Answer from the drawing. Dimensions are ordinates in mm from the lowest x, y and z of the part. A direction names the side the tool comes from. Round coordinates to 2 decimals unless told otherwise and drop trailing zeros. Order: outer loops, then holes, each group sorted by start corner. A loop starts at its lowest first (then second) coordinate and runs counter-clockwise, first axis right, second up.
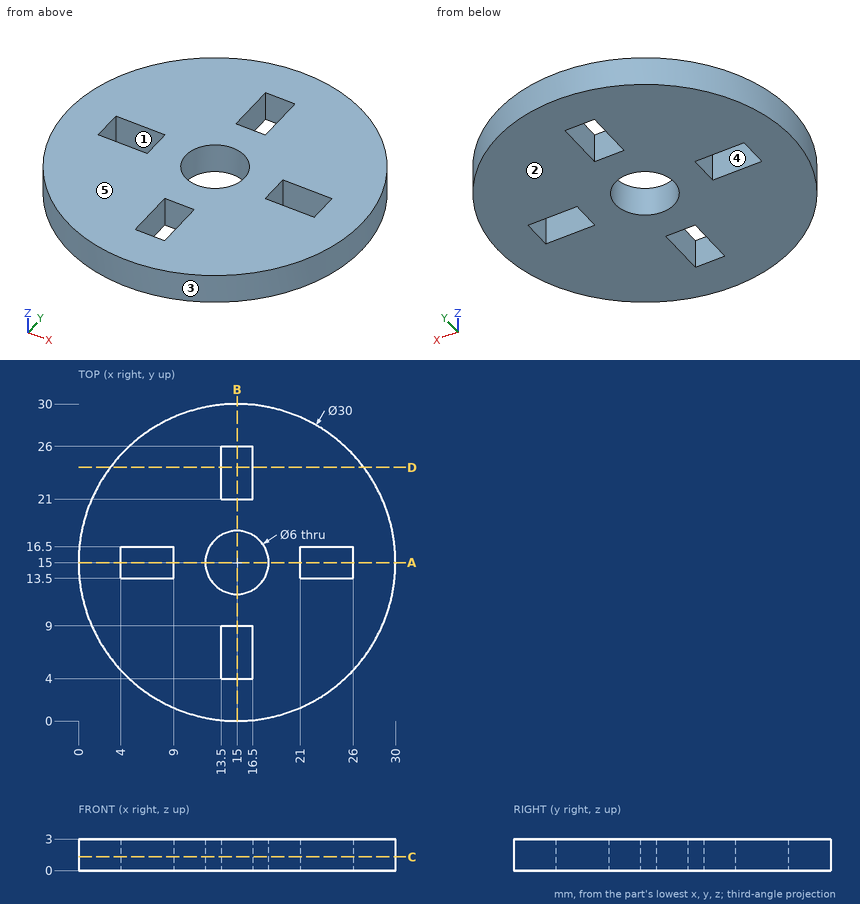
Q1. A cutting plane is placed at A-A, the plane y = 15. Give the vertices of the cut face in (x, z).
Outcome:
outline: (0, 0) - (4, 0) - (4, 3) - (0, 3) - close; (9, 0) - (12, 0) - (12, 3) - (9, 3) - close; (18, 0) - (21, 0) - (21, 3) - (18, 3) - close; (26, 0) - (30, 0) - (30, 3) - (26, 3) - close
Q2. A cutting plane is placed at C-C, the plane z = 1.3. Give the vertices of the cut face in (x, y), plus the area to 3 significant figures.
Outcome:
outline: circle Ø30 at (15, 15); hole (4, 13.5) - (9, 13.5) - (9, 16.5) - (4, 16.5) - close; hole circle Ø6 at (15, 15); hole (13.5, 4) - (16.5, 4) - (16.5, 9) - (13.5, 9) - close; hole (13.5, 21) - (16.5, 21) - (16.5, 26) - (13.5, 26) - close; hole (21, 13.5) - (26, 13.5) - (26, 16.5) - (21, 16.5) - close
area: 619 mm2
Q3. For the marked faces 1 and 2, determine the directions among +Z, -Z, +X, -X, +Y, -Y from which every point of the face is accessible in a straight line to the end or side of a thin tool.
Outcome:
face 1: +Z, -Z
face 2: -Z, +X, -X, +Y, -Y
Q4. Flat-ended cylindrical pins translate along their axes: pin 1 (0.9 mm diameter, centred on x = 7, z = 1.5, fed in from -Y); pin 2 (1.5 mm diameter, centred on x = 7.5, z = 1, fed in from +Y); pin 3 (1 mm diameter, centred on y = 6.5, z = 2, fed in from +X); pin 4 (5.5 mm diameter, centred on x = 15, y = 15, fed in from +Z). Find the tip coordinate at first contact, or state that the pin passes through.
Outcome:
pin 1: stops at y = 2.04
pin 2: stops at y = 28.4
pin 3: stops at x = 27.69
pin 4: passes through
Q5. For a pull along X with two mould halves and no side action, classify the marked faces 3, 4 and 5 as released by +X, released by -X, zero draft, split by the parting line, or undercut.
Outcome:
face 3: split by the parting line
face 4: undercut
face 5: zero draft
Q6. Straight lines are drawn through the part: probe 1 along Y at (x, z) = (15, 1.95); probe 2 along X at (y, z) = (14.25, 2.5); probe 3 along Y at (x, z) = (8, 2.25). For each, find the intervals that lie inside material, in ascending order.
Outcome:
probe 1: y = 0 to 4, 9 to 12, 18 to 21, 26 to 30
probe 2: x = 0.02 to 4, 9 to 12.1, 17.9 to 21, 26 to 29.98
probe 3: y = 1.73 to 13.5, 16.5 to 28.27
Q7. A cutting plane is placed at D-D, the plane y = 24. Give the vertices of the cut face in (x, z), plus the area to 3 significant figures.
Outcome:
outline: (3, 0) - (13.5, 0) - (13.5, 3) - (3, 3) - close; (16.5, 0) - (27, 0) - (27, 3) - (16.5, 3) - close
area: 63.0 mm2
